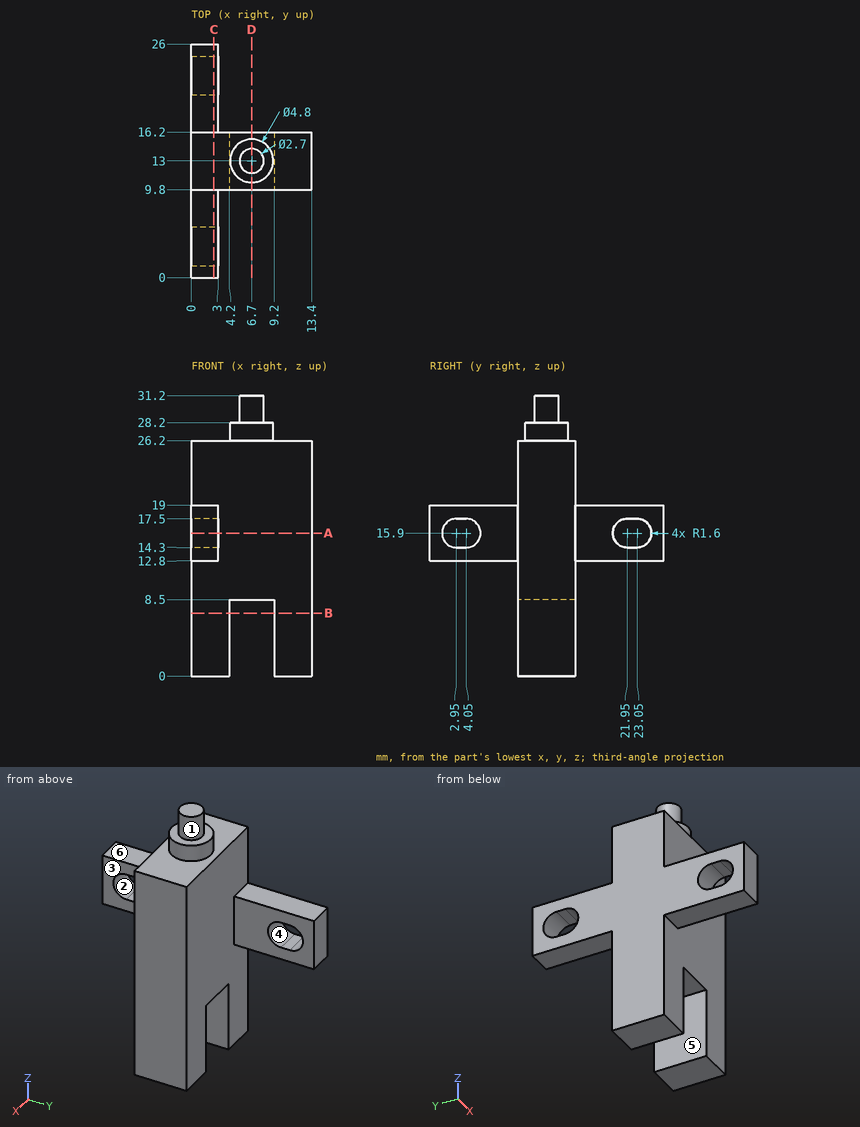
Here's the drawing with two shaded views (mm, measured from the low corner). I have some questions. A direction names the side the tool comes from. Coordinates: 2 decimals unless noted, no trailing zeros. Loops run counter-clockwise (first coordinate to the right, second up) from the corner with the lowest first, then second, coordinate; pieces in that order, holes last. Notation, with made-up numbers: M -0.75,54.25 L 4.25,54.25 A21 cw 4.25,90.25 Z; hole C 68,26 d11. An arc over 180 degrees is marked long. Put each result on its own line as item: value. Start each with the question number.
(1) Imagine slicing it at A-A on z = 15.9. List the corners of the cut face in (x, y) for me.
(2) Imagine slicing it at B-B on z = 7. List the corners of the cut face in (x, y) for me, and give its area (3 significant figures).
(3) Which directions (+Z, -Z, +X, -X, +Y, -Y) give clear straight access to the entire face, cutting with the end or side of a thin tool? Please do the marked faces 4, 5 and 6.
(4) Imagine slicing it at C-C on x = 2.5. List the corners of the cut face in (y, z) for me, and give its area (3 significant figures).
(5) Imagine slicing it at D-D on x = 6.7. List the corners of the cut face in (y, z) for me.
(6) We'd pull the mould along Y, two halves only. Please class the marked faces 1, 2 and 3: +Y half, -Y half, draft (parallel to the pull), parting line (faces both ways), or undercut.
(7) I need wall thicknesses on probe 1 along Y at (x, z) = (4.5, 12); probe 2 along Z at (x, y) = (1, 12.25); probe 3 along X at (y, z) = (9, 16). Which ranges of each line are inside material? Lowest first, please.
(8) Will these pins go through, and if not, where does the flat tip stop? pin 1 Ø4 at (x, z) = (10, 13) entering from +Y; pin 2 Ø1.5 at (x, y) = (1.5, 21.5) entering from +Z; pin 3 Ø1.5 at (x, y) = (7.5, 12.5) entering from -Z.
Worked answers:
1. outline: M 0,0 L 3,0 L 3,1.35 L 0,1.35 Z; M 0,5.65 L 3,5.65 L 3,9.8 L 13.4,9.8 L 13.4,16.2 L 3,16.2 L 3,20.35 L 0,20.35 Z; M 0,24.65 L 3,24.65 L 3,26 L 0,26 Z
2. outline: M 0,9.8 L 4.2,9.8 L 4.2,16.2 L 0,16.2 Z; M 9.2,9.8 L 13.4,9.8 L 13.4,16.2 L 9.2,16.2 Z
2. area: 53.8 mm2
3. face 4: +X, -X
3. face 5: -Z, +Y, -Y
3. face 6: +Z, +X, -X, -Y
4. outline: M 0,12.8 L 9.8,12.8 L 9.8,0 L 16.2,0 L 16.2,12.8 L 26,12.8 L 26,19 L 16.2,19 L 16.2,26.2 L 9.8,26.2 L 9.8,19 L 0,19 Z; hole M 2.95,14.3 L 4.05,14.3 A1.6 ccw 4.05,17.5 L 2.95,17.5 A1.6 ccw Z; hole M 21.95,14.3 L 23.05,14.3 A1.6 ccw 23.05,17.5 L 21.95,17.5 A1.6 ccw Z
4. area: 266 mm2
5. outline: M 9.8,8.5 L 16.2,8.5 L 16.2,26.2 L 15.4,26.2 L 15.4,28.2 L 14.35,28.2 L 14.35,31.2 L 11.65,31.2 L 11.65,28.2 L 10.6,28.2 L 10.6,26.2 L 9.8,26.2 Z
6. face 1: parting line
6. face 2: undercut
6. face 3: draft
7. probe 1: y = 9.8 to 16.2
7. probe 2: z = 0 to 26.2
7. probe 3: x = 0 to 3
8. pin 1: stops at y = 16.2
8. pin 2: stops at z = 19
8. pin 3: stops at z = 8.5
